from build123d import *

# Parameters (mm, degrees)
SKETCH1_R           = 7.5
SKETCH1_R_2         = 2.5
BOSS_EXTRUDE1_DEPTH = 15


with BuildPart() as part:
    # Sketch1 → Boss-Extrude1 (new body)
    with BuildSketch(Plane(origin=(0, 0, 0), x_dir=(0, 0, -1), z_dir=(1, 0, 0))):
        with BuildLine():
            Line((-13.228756555, -15), (13.228756555, -15))
            ThreePointArc((13.228756555, -15), (18.228756555, -8.228756555), (20, 0))
            Line((20, 0), (20, 35))
            Line((20, 35), (-20, 35))
            Line((-20, 35), (-20, 0))
            ThreePointArc((-20, 0), (-18.228756555, -8.228756555), (-13.228756555, -15))
        make_face()
        Circle(SKETCH1_R, mode=Mode.SUBTRACT)
        with Locations((16, 0)):
            Circle(SKETCH1_R_2, mode=Mode.SUBTRACT)
        with Locations((11.313708499, -11.313708499)):
            Circle(SKETCH1_R_2, mode=Mode.SUBTRACT)
        with Locations((-11.313708499, -11.313708499)):
            Circle(SKETCH1_R_2, mode=Mode.SUBTRACT)
        with Locations((-16, 0)):
            Circle(SKETCH1_R_2, mode=Mode.SUBTRACT)
        with Locations((-11.313708499, 11.313708499)):
            Circle(SKETCH1_R_2, mode=Mode.SUBTRACT)
        with Locations((11.313708499, 11.313708499)):
            Circle(SKETCH1_R_2, mode=Mode.SUBTRACT)
        with BuildLine():
            Line((-12.25, 23), (-12.25, 27))
            ThreePointArc((-12.25, 27), (-10, 29.25), (-7.75, 27))
            Line((-7.75, 27), (-7.75, 23))
            ThreePointArc((-7.75, 23), (-10, 20.75), (-12.25, 23))
        make_face(mode=Mode.SUBTRACT)
        with BuildLine():
            Line((12.25, 23), (12.25, 27))
            ThreePointArc((12.25, 27), (10, 29.25), (7.75, 27))
            Line((7.75, 27), (7.75, 23))
            ThreePointArc((7.75, 23), (10, 20.75), (12.25, 23))
        make_face(mode=Mode.SUBTRACT)
    extrude(amount=BOSS_EXTRUDE1_DEPTH)


solid = part.part
Verification items for the finished model (mm, model axes). A direction names the side the tool comes from. Coordinates: 2 decimals unless noted, no trailing zeros. Order: outer loops, then holes, each group sorted by start corner. A loop starts at its lowest first (then second) coordinate and runs counter-clockwise, first axis right, second up. Notation, with made-up numbers: (8.25, 71) -> (34.25, 71) arc R30 cw to (34.25, 95) -> close; hole circle Ø6 at (36, 43.5). An arc over 180 degrees is marked (long way). Put each result on its own line as item: value. Start each with the question number.
1. Access from +Z, -Z, +X, -X, +Y, -Y to the whole of each face (thin tool, end or side, straight path). Record for faces 1 (the flat face through (7, 17, -20)), 2 (the cylindrical face through (7.4, 20.75, -9.95)).
2. Material ranges on L1, parallel to Z at x = 6.5, y = 25; L2, parallel to Z at x = 1.25, y = -12.5; L3, parallel to Y at x = 3.75, z = 0, recorded low to high. Write a range as [from, to].
3. Cross-section at A-A, the plane z = 0. Record the boundary of the cut face in (x, y).
4. Mould release check, pull along Y, two halves, no side actions. Record for faces 3 (the flat face through (0, 10, 0)), 4 (the flat face through (7, 25, 7.75)), 5 (the cylindrical face through (7.4, -8.34, -18.18)), 6 (the flat face through (7, 35, 0)): released by +Y, released by -Y, zero draft, split by the parting line, or undercut.
5. Cross-section at B-B, the plane y = 9.5. Record the boundary of the cut face in (x, z).
6. Cross-section at C-C, the plane z = -16. Record the boundary of the cut face in (x, y).
7. Go/stop test with flat-tipped pins: pin 1 Ø4 at (y, z) = (-11.31, -11.31) entering from -X; pin 2 Ø8 at (y, z) = (11.31, -11.31) entering from -X. Record where each tip stops, or that it passes through.
8. Cross-section at D-D, the plane x = 12.5. Count the separate pieces of the cut face and the enclosed holes in it, then the cut area to 3 significant figures.
Computed:
1. face 1: -Z, +X, -X, +Y, -Y
1. face 2: +X, -X
2. L1: [-20, -12.25], [-7.75, 7.75], [12.25, 20]
2. L2: [-15.61, -13.51], [-9.11, 9.11], [13.51, 15.61]
2. L3: [-15, -7.5], [7.5, 35]
3. outline: (0, -15) -> (15, -15) -> (15, -7.5) -> (0, -7.5) -> close; (0, 7.5) -> (15, 7.5) -> (15, 35) -> (0, 35) -> close
4. face 3: zero draft
4. face 4: undercut
4. face 5: released by -Y
4. face 6: released by +Y
5. outline: (0, -20) -> (15, -20) -> (15, -13.03) -> (0, -13.03) -> close; (0, -9.59) -> (15, -9.59) -> (15, 9.59) -> (0, 9.59) -> close; (0, 13.03) -> (15, 13.03) -> (15, 20) -> (0, 20) -> close
6. outline: (0, -12) -> (15, -12) -> (15, -2.5) -> (0, -2.5) -> close; (0, 2.5) -> (15, 2.5) -> (15, 35) -> (0, 35) -> close
7. pin 1: through
7. pin 2: x = 0
8. separate pieces: 1
8. enclosed holes: 9
8. area: 1,580 mm2
